```python
from build123d import *

# Parameters (mm, degrees)
F0_W     = 65
F0_H     = 65
F1_DEPTH = 30
F2_T     = -5


with BuildPart() as f1:
    # F0 (on Top) → F1 (new body, symmetric)
    with BuildSketch(Plane.XY):
        with Locations((2.5, 0)):
            Rectangle(F0_W, F0_H)
    extrude(amount=F1_DEPTH, both=True)

    # F2
    f2_openings = [f1.faces().sort_by_distance(p)[0] for p in [
        (2.5, 32.5, 0),
    ]]
    offset(amount=F2_T, openings=f2_openings)


solid = f1.part
```
For this review, take the finished solid that the model builds, in its own axes (mm). A direction names the side the tool comes from. Round coordinates to 2 decimals unless told otherwise and drop trailing zeros. Write each loop counter-clockwise with the first axis right and the second up, starting at its lowest first coordinate (ties: lowest second). Pieces come first, ordered by that corner, then holes. Notation, with made-up numbers: (10, 8) - (15, 8) arc R34 cw to (15, 43) - close; hole circle Ø5 at (71, 53). An arc over 180 degrees is marked (long way). Answer as a JSON object with one key per item and string values.
1. Tool access review of faces 1 (the face through (2, -32.5, 0)), 2 (the face through (2, -27.5, 0)): name each direction out of +Z, -Z, +X, -X, +Y, -Y from which nothing blocks a thin tool from reaching the whole face with its end or side.
Response values:
{"face 1": "+Z, -Z, +X, -X, -Y", "face 2": "+Y"}
2. For pin 1 Ø2 at (x, z) = (-3.5, -11) entering from +Y, flat-tipped, find the tip position at first contact; note if it passes through.
Response values:
{"pin 1": "stops at y = -27.5"}
3. We need section B-B on x = 16. Give the boundary of the cut face in (y, z).
Response values:
{"outline": "(-32.5, -30) - (32.5, -30) - (32.5, -25) - (-27.5, -25) - (-27.5, 25) - (32.5, 25) - (32.5, 30) - (-32.5, 30) - close"}
4. To check wall thickness, follow line 1 along Z through (x, y) = (-13.5, 21.5); line 2 along X through (y, z) = (4, 14); line 3 along Y through (x, z) = (-10, -5). State the ranges of each line that lie inside material, in increasing order.
Response values:
{"line 1": "z = -30 to -25, 25 to 30", "line 2": "x = -30 to -25, 30 to 35", "line 3": "y = -32.5 to -27.5"}
5. We need section C-C on z = 0. Give the boundary of the cut face in (x, y), then the cut area to 3 significant figures.
Response values:
{"outline": "(-30, -32.5) - (35, -32.5) - (35, 32.5) - (30, 32.5) - (30, -27.5) - (-25, -27.5) - (-25, 32.5) - (-30, 32.5) - close", "area": "925 mm2"}
6. We need section A-A on y = -1.5. Give the boundary of the cut face in (x, z), then the cut area to 3 significant figures.
Response values:
{"outline": "(-30, -30) - (35, -30) - (35, 30) - (-30, 30) - close; hole (-25, -25) - (30, -25) - (30, 25) - (-25, 25) - close", "area": "1,150 mm2"}
